Read the model definition and answer for the solid it produces. Units are mm, in the model's axes. Coordinates: 2 decimals unless noted, no trailing zeros. Order: outer loops, then holes, each group sorted by start corner. A loop starts at its lowest first (then second) coordinate and runs counter-clockwise, first axis right, second up.
```python
from build123d import *

# Parameters (mm, degrees)
SKETCH1_W           = 10
SKETCH1_H           = 3.175
SKETCH1_W_2         = 3.175
SKETCH1_H_2         = 50
BOSS_EXTRUDE1_DEPTH = 3.175


with BuildPart() as part:
    # Sketch1 → Boss-Extrude1 (new body)
    with BuildSketch(Plane(origin=(0, -2.422329102, -69.308356399), x_dir=(-1, 0, 0), z_dir=(0, -0.03492870325036369, -0.9993898066766782))):
        with BuildLine():
            Line((-5, 79.214647081), (-1.5875, 79.214647081))
            Line((-1.5875, 79.214647081), (-1.5875, 129.214647081))
            Line((-1.5875, 129.214647081), (-1.5875, 204.214647081))
            Line((-1.5875, 204.214647081), (-0.8375, 204.214647081))
            Line((-0.8375, 204.214647081), (-0.8375, 229.214647081))
            Line((-0.8375, 229.214647081), (-1.5875, 229.214647081))
            Line((-1.5875, 229.214647081), (-1.5875, 304.214647081))
            Line((-1.5875, 304.214647081), (-0.8375, 304.214647081))
            Line((-0.8375, 304.214647081), (-0.8375, 329.214647081))
            Line((-0.8375, 329.214647081), (-3.3375, 329.214647081))
            ThreePointArc((-3.3375, 329.214647081), (-13.715159098, 202.525816485), (-44.57145678, 79.214647081))
            Line((-44.57145678, 79.214647081), (-38.57145678, 79.214647081))
            Line((-38.57145678, 79.214647081), (-28.57145678, 79.214647081))
            Line((-28.57145678, 79.214647081), (-5, 79.214647081))
        make_face()
        with BuildLine():
            ThreePointArc((44.57145678, 79.214647081), (13.715159098, 202.525816485), (3.3375, 329.214647081))
            Line((3.3375, 329.214647081), (0.8375, 329.214647081))
            Line((0.8375, 329.214647081), (0.8375, 304.214647081))
            Line((0.8375, 304.214647081), (1.5875, 304.214647081))
            Line((1.5875, 304.214647081), (1.5875, 229.214647081))
            Line((1.5875, 229.214647081), (0.8375, 229.214647081))
            Line((0.8375, 229.214647081), (0.8375, 204.214647081))
            Line((0.8375, 204.214647081), (1.5875, 204.214647081))
            Line((1.5875, 204.214647081), (1.5875, 129.214647081))
            Line((1.5875, 129.214647081), (1.5875, 79.214647081))
            Line((1.5875, 79.214647081), (5, 79.214647081))
            Line((5, 79.214647081), (28.57145678, 79.214647081))
            Line((28.57145678, 79.214647081), (38.57145678, 79.214647081))
            Line((38.57145678, 79.214647081), (44.57145678, 79.214647081))
        make_face()
        Polygon((5, 76.039647081), (5, 79.214647081), (1.5875, 79.214647081), (-1.5875, 79.214647081), (-5, 79.214647081), (-5, 76.039647081), align=None)
        with Locations((33.57145678, 77.627147081)):
            Rectangle(SKETCH1_W, SKETCH1_H)
        with Locations((0, 104.214647081)):
            Rectangle(SKETCH1_W_2, SKETCH1_H_2)
        with Locations((-33.57145678, 77.627147081)):
            Rectangle(SKETCH1_W, SKETCH1_H)
    extrude(amount=BOSS_EXTRUDE1_DEPTH)


solid = part.part
```
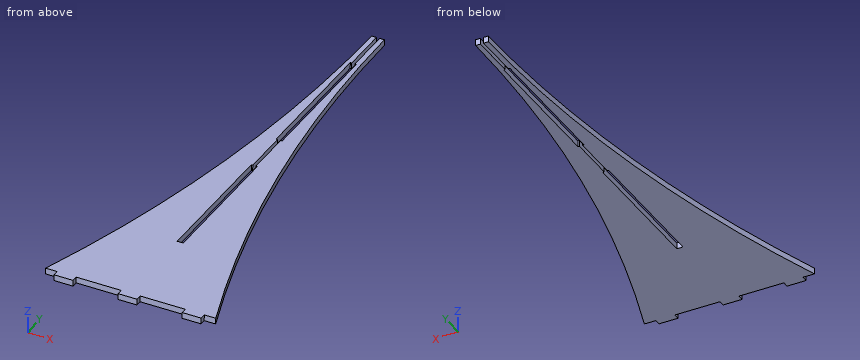
1) Flat-ended cylindrical pins translate along their axes: pin 1 Ø2.5 at (y, z) = (75, -73) entering from -X; pin 2 Ø4 at (x, z) = (-16.5, -76.5) entering from -Y; pin 3 Ø3 at (y, z) = (213, -79) entering from +X; pin 4 Ø3.5 at (y, z) = (76, -73.5) entering from +X. Find the tip coordinate at first contact, or state that the pin passes through.
A:
pin 1: stops at x = -38.57
pin 2: stops at y = 76.63
pin 3: stops at x = 11.89
pin 4: stops at x = 44.57
2) A cutting plane is placed at B-B, the plane x = 23.5. Determine the outline of the cut face in (y, z).
A:
outline: (76.63, -75.25) - (150.56, -77.83) - (150.67, -74.66) - (76.74, -72.08) - close
3) A cutting plane is placed at A-A, the plane x = -22. Determine the outline of the cut face in (y, z), and give its area (3 significant figures).
A:
outline: (76.63, -75.25) - (157.15, -78.06) - (157.26, -74.89) - (76.74, -72.08) - close
area: 256 mm2
4) Straight lines are drawn through the part: line 1 (Y direction, x = 0, z = -74); line 2 (X direction, y = 169, z = -77.25); line 3 (Z direction, x = 2.5, y = 282). For each, find the intervals that lie inside material, in ascending order.
A:
line 1: y = 73.5 to 126.71
line 2: x = -19.46 to -1.59, 1.59 to 19.46
line 3: z = -82.43 to -79.25
